Check sheet for the modelled part. Datum: model origin and axes. Units: mm. Face numbers are marked on the shaded views. A direction names the side the tool comes from. Round coordinates to 2 decimals unless told otherwise and drop trailing zeros. Order: outer loops, then holes, each group sorted by start corner. A loop starts at its lowest first (then second) coordinate and runs counter-clockwise, first axis right, second up.
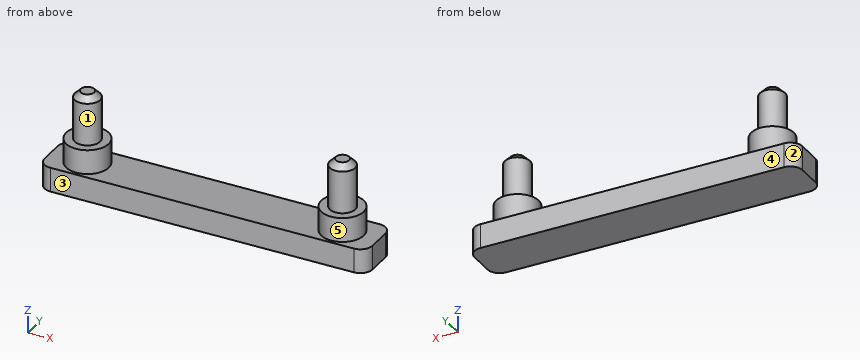
```python
from build123d import *

# Parameters (mm, degrees)
F0_W     = 27
F0_H     = 4
F1_DEPTH = 2
F2_R     = 1.05
F3_DEPTH = 6
F4_SIZE  = 0.5
F5_R     = 1
F6_R     = 1.75
F7_DEPTH = 2


with BuildPart() as f1:
    # F0 (on Top) → F1 (new body)
    with BuildSketch(Plane.XY):
        Rectangle(F0_W, F0_H)
    extrude(amount=F1_DEPTH)

    # F2 (on face) → F3 (join)
    with BuildSketch(Plane.XY.offset(2)):
        with Locations((-10.5, 0)):
            Circle(F2_R)
        with BuildLine():
            ThreePointArc((11.55, 0), (10.5, 1.05), (9.45, 0))
            ThreePointArc((9.45, 0), (10.5, -1.05), (11.55, 0))
        make_face()
    extrude(amount=F3_DEPTH)

    # F4
    f4_edges = [f1.edges().sort_by_distance(p)[0] for p in [
        (-11.55, 0, 8),
        (11.55, 0, 8),
    ]]
    chamfer(f4_edges, length=F4_SIZE)

    # F5
    f5_edges = [f1.edges().sort_by_distance(p)[0] for p in [
        (-13.5, -2, 1),
        (-13.5, 2, 1),
        (13.5, 2, 1),
        (13.5, -2, 1),
    ]]
    fillet(f5_edges, radius=F5_R)

    # F6 (on face) → F7 (join)
    with BuildSketch(Plane.XY.offset(2)):
        with Locations((-10.5, 0)):
            Circle(F6_R)
        with Locations((10.5, 0)):
            Circle(F6_R)
    extrude(amount=F7_DEPTH)


solid = f1.part
```
Item 1: Scan lines: line 1 along X through (y, z) = (0.1, 3); line 2 along Z through (x, y) = (-9, -0.2); line 3 along Z through (x, y) = (6, 0.8). Record each from-to range of solid material in increasing order.
Answer:
line 1: x = -12.25 to -8.75, 8.75 to 12.25
line 2: z = 0 to 4
line 3: z = 0 to 2
Item 2: Sectioned sample at B-B (z = 2.25). Record the cut outline in (x, y), and give its area (3 significant figures).
Answer:
outline: circle Ø3.5 at (-10.5, 0); circle Ø3.5 at (10.5, 0)
area: 19.2 mm2
Item 3: Access from +Z, -Z, +X, -X, +Y, -Y to the whole of each face (thin tool, end or side, straight path). Record for the marked faces 4 and 5.
Answer:
face 4: +Z, -Z, +X, -X, +Y
face 5: +Z
Item 4: Go/stop test with flat-tipped pins: P1, Ø4, axis at x = -9.5, z = 6.5, coming from the +Y side; P2, Ø1, axis at x = -9.5, y = 0.5, coming from the +Z side; P3, Ø2, axis at x = -9.5, y = 1.5, coming from the +Z side. Record where each tip stops, or that it passes through.
Answer:
P1: stops at y = 1.05
P2: stops at z = 7.93
P3: stops at z = 7.75
Item 5: Sectioned sample at D-D (z = 5). Record the cut outline in (x, y), and give its area (3 significant figures).
Answer:
outline: circle Ø2.1 at (-10.5, 0); circle Ø2.1 at (10.5, 0)
area: 6.93 mm2
Item 6: Sectioned sample at A-A (y = 0). Record the cut outline in (x, z).
Answer:
outline: (-13.5, 0) - (13.5, 0) - (13.5, 2) - (12.25, 2) - (12.25, 4) - (11.55, 4) - (11.55, 7.5) - (11.05, 8) - (9.95, 8) - (9.45, 7.5) - (9.45, 4) - (8.75, 4) - (8.75, 2) - (-8.75, 2) - (-8.75, 4) - (-9.45, 4) - (-9.45, 7.5) - (-9.95, 8) - (-11.05, 8) - (-11.55, 7.5) - (-11.55, 4) - (-12.25, 4) - (-12.25, 2) - (-13.5, 2) - close
Item 7: Sectioned sample at C-C (x = 10.5). Record the cut outline in (y, z).
Answer:
outline: (-2, 0) - (2, 0) - (2, 2) - (1.75, 2) - (1.75, 4) - (1.05, 4) - (1.05, 7.5) - (0.55, 8) - (-0.55, 8) - (-1.05, 7.5) - (-1.05, 4) - (-1.75, 4) - (-1.75, 2) - (-2, 2) - close
Item 8: Release check for a two-part mould opening along X. For the marked faces 1, 2 and 3 record: released by +X, released by -X, zero draft, split by the parting line, or undercut.
Answer:
face 1: undercut
face 2: released by -X
face 3: zero draft
